Study the drawing (mm; zero at the part's minimum x, y, z) and answer. Coordinates: 2 decimals unless noted, no trailing zeros. Order: outer loops, then holes, each group sorted by start corner. A loop starts at its lowest first (then second) coordinate and runs counter-clockwise, first axis right, second up. Notation, with made-up numbers: (6.25, 46) -> (61.25, 46) arc R8 cw to (61.25, 53) -> close; hole circle Ø6 at (11, 75.25). An arc over 180 degrees is marked (long way). Write each question's results on one line, items separated by ' | '. Start each with the question number.
(1) A straight line is drawn through the part: L1, parallel to X at y = 8.5, z = 54.5. Find the intervals that lie inside material, in ascending order.
(2) Given pin 1 (25 mm diameter, centred on x = 1368.5, y = 45, fed in from +Z); pin 2 (15 mm diameter, centred on x = 1370.5, z = 43, fed in from -Y); pin 3 (25 mm diameter, centred on x = 1368.5, y = 45, fed in from -Z), each flat-ended and moving along its own axis, determine where each tip first touches the part or whether it passes through.
(3) The part is cut by section B-B, the plane y = 35. Give the vertices of the cut face in (x, z).
(4) The part is cut by section A-A, the plane z = 24. Give the vertices of the cut face in (x, y).
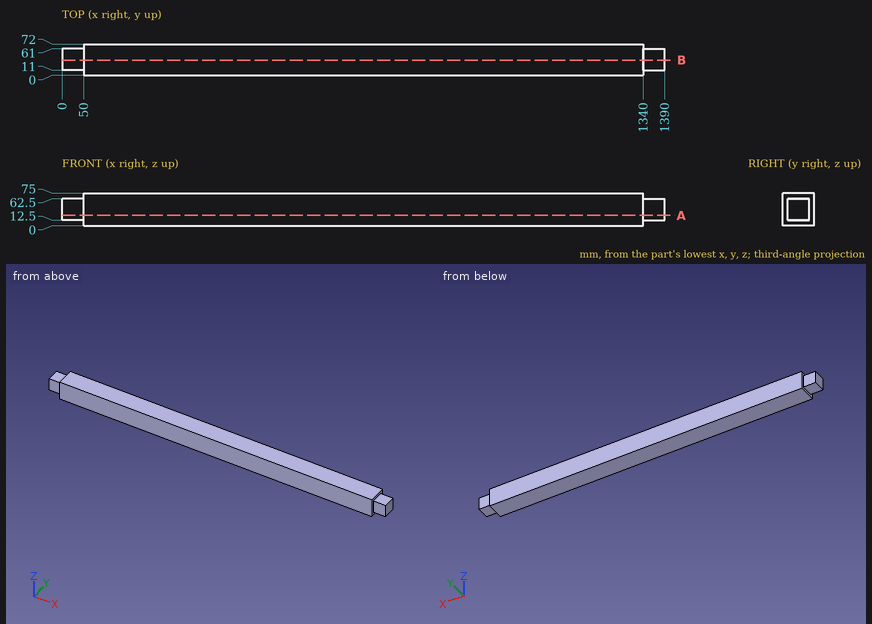
Established:
1) L1: x = 50 to 1340
2) pin 1: stops at z = 62.5 | pin 2: stops at y = 11 | pin 3: stops at z = 12.5
3) outline: (0, 12.5) -> (50, 12.5) -> (50, 0) -> (1340, 0) -> (1340, 12.5) -> (1390, 12.5) -> (1390, 62.5) -> (1340, 62.5) -> (1340, 75) -> (50, 75) -> (50, 62.5) -> (0, 62.5) -> close
4) outline: (0, 11) -> (50, 11) -> (50, 0) -> (1340, 0) -> (1340, 11) -> (1390, 11) -> (1390, 61) -> (1340, 61) -> (1340, 72) -> (50, 72) -> (50, 61) -> (0, 61) -> close
